Autodesk Inventor part; units mm, degrees
ref_plane "YZ Plane" through (0, 0, 0) normal (1, 0, 0) x (0, 1, 0)
ref_plane "XZ Plane" through (0, 0, 0) normal (0, 1, 0) x (-1, 0, 0)
ref_plane "XY Plane" through (0, 0, 0) normal (0, 0, 1) x (1, 0, 0)
sketch "Sketch1" plane through (0, 0, 0) normal (0, 1, 0) x (-1, 0, 0)
  line L0 (-13.5, -12.4952) -> (9.75, -12.4952)
  line L1 (9.75, -12.4952) -> (9.75, 12.4952)
  line L2 (9.75, 12.4952) -> (-13.5, 12.4952)
  line L3 (-13.5, 12.4952) -> (-13.5, -12.4952)
  circle A0 centre (-7.5, 0) radius 4
  circle A1 centre (3.75, -6.4952) radius 4
  circle A2 centre (3.75, 6.4952) radius 4
  line L4 (-2.75, -1.5877) -> (-2.75, 1.5877)
  line L5 (-2.75, 1.5877) -> (0, 3.1754)
  line L6 (0, 3.1754) -> (2.75, 1.5877)
  line L7 (2.75, 1.5877) -> (2.75, -1.5877)
  line L8 (2.75, -1.5877) -> (0, -3.1754)
  line L9 (0, -3.1754) -> (-2.75, -1.5877)
  circle A3 centre (0, 0) radius 7.5 construction
  dimension "d11" = 15
  dimension "d2" = 8
  dimension "d6" = 360
  dimension "d8" = 6
  dimension "d9" = 6
  dimension "d10" = 5.5
  dimension "d12" = 6
  dimension "d13" = 6
extrude "Extrusion1" add sketch "Sketch1" along normal blind 3 contours L3 L2 L1 L0 | L4 L5 L6 L7 L8 L9
sketch "Sketch2" plane through (0, 3, 0) normal (0, 1, 0) x (1, 0, 0)
  circle A0 centre (-3.75, -6.4952) radius 4
  circle A1 centre (-3.75, 6.4952) radius 4
  circle A2 centre (7.5, 0) radius 4
  line L0 (13.5, 12.4952) -> (-9.75, 12.4952)
  line L1 (-9.75, 12.4952) -> (-9.75, -12.4952)
  line L2 (-9.75, -12.4952) -> (13.5, -12.4952)
  line L3 (13.5, -12.4952) -> (13.5, 12.4952)
  circle A3 centre (0, 0) radius 2.5
  dimension "d16" = 5
extrude "Extrusion2" add sketch "Sketch2" along normal blind 0.5 contours A0 | A1 | A2 | L3 L2 L1 L0
sketch "Sketch3" plane through (0, 0, 0) normal (0, -1, 0) x (1, 0, 0)
  circle A0 centre (-3.75, 6.4952) radius 4
  circle A1 centre (-3.75, -6.4952) radius 4
  circle A2 centre (7.5, 0) radius 4
  line L0 (13.5, -12.4952) -> (-9.75, -12.4952)
  line L1 (13.5, 12.4952) -> (13.5, -12.4952)
  line L2 (-9.75, 12.4952) -> (13.5, 12.4952)
  line L3 (-9.75, -12.4952) -> (-9.75, 12.4952) construction
  line L4 (-1.5, 12.4952) -> (13.5, 3.4952)
  line L5 (13.5, 12.4952) -> (13.5, -12.4952)
  line L6 (13.5, -3.4952) -> (-1.5, -12.4952)
  circle A3 centre (0, 0) radius 2.5
  dimension "d19" = 9
  dimension "d20" = 9
  dimension "d21" = 15
  dimension "d22" = 15
extrude "Extrusion3" cut sketch "Sketch3" against normal through all contours L4 L2 L1 | L0 L6 L1 | A3
properties part number "30_Cube_Z_Focus_Drylin_NEMA_slide_part1"
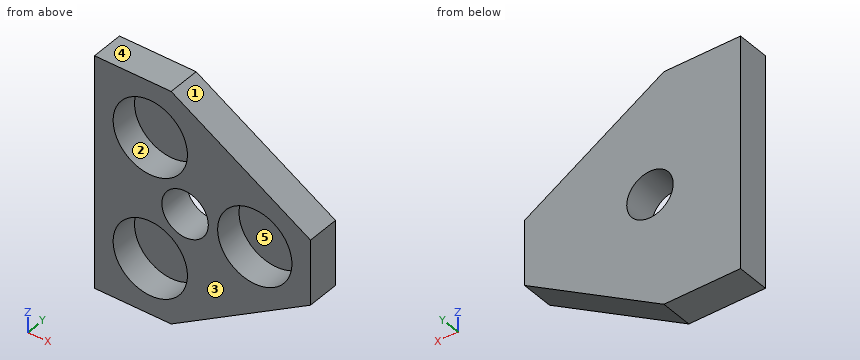
Geometry: final body of the model. Coordinates: model frame, mm. Face numbers are marked on the shaded views. A direction names the side the tool comes from. Give positions to 0.01 mm unless a question says otherwise; leave off trailing zeros. Order: outer loops, then holes, each group sorted by start corner. A loop starts at its lowest first (then second) coordinate and runs counter-clockwise, first axis right, second up. Notation, with made-up numbers: (21, 23.5) -> (56, 23.5) arc R21 cw to (56, 61.5) -> close; hole circle Ø6 at (61, 78). An arc over 180 degrees is marked (long way). Put each result on its own line as item: value.
Q1. Material intervals for L1, parallel to Z at x = -3.75, y = 0.7; L2, parallel to X at y = 1.4, z = -2.25; L3, parallel to X at y = 2.35, z = -0.25, sorted ascending.
Here are the results:
L1: z = -12.5 to -10.5, -2.5 to 2.5, 10.5 to 12.5
L2: x = -9.75 to -1.09, 1.09 to 4.19, 10.81 to 13.5
L3: x = -9.75 to -2.49, 2.49 to 3.51, 11.49 to 13.5
Q2. Draft query along X for the marked faces 1, 2 and 3. Return one class per face: released by +X, released by -X, zero draft, split by the parting line, or undercut.
Here are the results:
face 1: released by +X
face 2: undercut
face 3: zero draft
Q3. Section A-A, the plane z = 0. Return loops of the section in (x, y).
Here are the results:
outline: (-9.75, 0) -> (-2.5, 0) -> (-2.5, 3.5) -> (-9.75, 3.5) -> close; (2.5, 0) -> (3.5, 0) -> (3.5, 3) -> (11.5, 3) -> (11.5, 0) -> (13.5, 0) -> (13.5, 3.5) -> (2.5, 3.5) -> close
Q4. Pin query (flat end, axial travel): pin 1 (5 mm diameter, centred on x = -1.5, z = 10, fed in from -Y); pin 2 (2.5 mm diameter, centred on x = -4, z = -4.5, fed in from -Y). Return the tip coordinate at first contact, or that it passes through.
Here are the results:
pin 1: stops at y = 0
pin 2: stops at y = 3
Q5. Section B-B, the plane x = -3.75. Return loops of the section in (y, z).
Here are the results:
outline: (0, -12.5) -> (3.5, -12.5) -> (3.5, 12.5) -> (0, 12.5) -> (0, 10.5) -> (3, 10.5) -> (3, 2.5) -> (0, 2.5) -> (0, -2.5) -> (3, -2.5) -> (3, -10.5) -> (0, -10.5) -> close
Q6. Section C-C, the plane y = 1.7. Return loops of the section in (x, z), then the cut area to 3 significant figures.
Here are the results:
outline: (-9.75, -12.5) -> (-1.5, -12.5) -> (13.5, -3.5) -> (13.5, 3.5) -> (-1.5, 12.5) -> (-9.75, 12.5) -> close; hole circle Ø8 at (-3.75, -6.5); hole circle Ø8 at (-3.75, 6.5); hole circle Ø5 at (0, 0); hole circle Ø8 at (7.5, 0)
area: 276 mm^2
Q7. Reachability of the marked faces 4 and 5 from +Z, -Z, +X, -X, +Y, -Y: full face, straight path, thin tool, end or side. Return the list, or none.
Here are the results:
face 4: +Z, +X, -X, +Y, -Y
face 5: -Y
Q8. Section D-D, the plane x = -0.25. Return loops of the section in (y, z), then the cut area to 3 significant figures.
Here are the results:
outline: (0, -11.75) -> (3.5, -11.75) -> (3.5, -2.49) -> (0, -2.49) -> (0, -4.56) -> (3, -4.56) -> (3, -8.43) -> (0, -8.43) -> close; (0, 2.49) -> (3.5, 2.49) -> (3.5, 11.75) -> (0, 11.75) -> (0, 8.43) -> (3, 8.43) -> (3, 4.56) -> (0, 4.56) -> close
area: 41.6 mm^2
